from build123d import *

# Parameters (mm, degrees)
BOSS_EXTRUDE3_DEPTH  = 10
SKETCH2_W            = 34
SKETCH2_H            = 17
SKETCH2_W_2          = 30
SKETCH2_H_2          = 13
BOSS_EXTRUDE4_DEPTH  = 5
SKETCH3_W            = 50
SKETCH3_H            = 120
BOSS_EXTRUDE5_DEPTH  = 50
CUT_EXTRUDE2_DEPTH   = 50
SKETCH5_W            = 50
SKETCH5_H            = 180
BOSS_EXTRUDE6_DEPTH  = 50
CUT_EXTRUDE3_DEPTH   = 346.480399988
SKETCH7_W            = 5
SKETCH7_H            = 300
BOSS_EXTRUDE7_DEPTH  = 70
SKETCH9_W            = 34
SKETCH9_H            = 17
SKETCH9_W_2          = 30
SKETCH9_H_2          = 13
BOSS_EXTRUDE8_DEPTH  = 5
SKETCH10_W           = 55.647662557
SKETCH10_H           = 60
BOSS_EXTRUDE9_DEPTH  = 35
SKETCH13_W           = 13
SKETCH13_H           = 30
SKETCH13_W_2         = 8.592805021
SKETCH13_H_2         = 26
BOSS_EXTRUDE11_DEPTH = 5
SKETCH14_R           = 8
BOSS_EXTRUDE12_DEPTH = 27
SKETCH16_R           = 8
BOSS_EXTRUDE13_DEPTH = 27
SKETCH17_R           = 12
BOSS_EXTRUDE14_DEPTH = 5
SKETCH18_R           = 12
BOSS_EXTRUDE15_DEPTH = 5


with BuildPart() as part:
    # Sketch1 → Boss-Extrude3 (new body)
    with BuildSketch(Plane(origin=(0, 0, 0), x_dir=(1, 0, 0), z_dir=(0, 1, 0))):
        Polygon((-100.4558, 255.209143206), (299.5442, 255.209143206), (299.5442, 0.092543206), (229.0884, 0.092543206), (229.0884, -44.790856794), (-30, -44.790856794), (-30, 0.092543206), (-100.4558, 0.092543206), align=None)
    extrude(amount=BOSS_EXTRUDE3_DEPTH)

    # Sketch2 → Boss-Extrude4 (add)
    # profile 1 of 2: a face of its own
    with BuildSketch(Plane(origin=(0, 10, 0), x_dir=(1, 0, 0), z_dir=(0, 1, 0))):
        with Locations((-13, -22.349156794)):
            Rectangle(SKETCH2_W, SKETCH2_H)
        with Locations((-13, -22.349156794)):
            Rectangle(SKETCH2_W_2, SKETCH2_H_2, mode=Mode.SUBTRACT)
    # profile 2 of 2: a face of its own
    with BuildSketch(Plane(origin=(0, 10, 0), x_dir=(1, 0, 0), z_dir=(0, 1, 0))):
        with Locations((212.0884, -22.349156794)):
            Rectangle(SKETCH2_W, SKETCH2_H)
        with Locations((212.0884, -22.349156794)):
            Rectangle(SKETCH2_W_2, SKETCH2_H_2, mode=Mode.SUBTRACT)
    extrude(amount=BOSS_EXTRUDE4_DEPTH)

    # Sketch3 → Boss-Extrude5 (add)
    with BuildSketch(Plane(origin=(0, 10, 0), x_dir=(1, 0, 0), z_dir=(0, 1, 0))):
        with Locations((99.5442, 15.209143206)):
            Rectangle(SKETCH3_W, SKETCH3_H)
    extrude(amount=BOSS_EXTRUDE5_DEPTH)

    # Sketch4 → Cut-Extrude2 (cut)
    with BuildSketch(Plane(origin=(124.5442, 0, 0), x_dir=(0, 0, -1), z_dir=(1, 0, 0))):
        Polygon((-44.790856794, 60), (75.209143206, 60), (-44.790856794, 0), align=None)
    extrude(amount=-CUT_EXTRUDE2_DEPTH, mode=Mode.SUBTRACT)

    # Sketch5 → Boss-Extrude6 (add)
    with BuildSketch(Plane(origin=(0, 10, 0), x_dir=(1, 0, 0), z_dir=(0, 1, 0))):
        with Locations((99.5442, 165.209143206)):
            Rectangle(SKETCH5_W, SKETCH5_H)
    extrude(amount=BOSS_EXTRUDE6_DEPTH)

    # Sketch6 → Cut-Extrude3 (cut, through all)
    with BuildSketch(Plane(origin=(124.5442, 0, 0), x_dir=(0, 0, -1), z_dir=(1, 0, 0))):
        Polygon((75.209143206, 60), (255.209143206, 60), (255.209143206, 30), align=None)
    extrude(amount=-CUT_EXTRUDE3_DEPTH, mode=Mode.SUBTRACT)

    # Sketch7 → Boss-Extrude7 (add)
    with BuildSketch(Plane(origin=(0, 0, 0), x_dir=(1, 0, 0), z_dir=(0, 1, 0))):
        with Locations((72.0442, 105.209143206)):
            Rectangle(SKETCH7_W, SKETCH7_H)
        Polygon((129.5442, 255.209143206), (124.5442, 255.209143206), (124.5442, -44.790856794), (164.5442, -44.790856794), (164.5442, 0), (129.5442, 0), align=None)
    extrude(amount=BOSS_EXTRUDE7_DEPTH)

    # Sketch9 → Boss-Extrude8 (add)
    with BuildSketch(Plane(origin=(0, 70, 0), x_dir=(1, 0, 0), z_dir=(0, 1, 0))):
        with Locations((141.5442, -24.790856794)):
            Rectangle(SKETCH9_W, SKETCH9_H)
        with Locations((141.5442, -24.790856794)):
            Rectangle(SKETCH9_W_2, SKETCH9_H_2, mode=Mode.SUBTRACT)
    extrude(amount=BOSS_EXTRUDE8_DEPTH)

    # Sketch10 → Boss-Extrude9 (add)
    with BuildSketch(Plane(origin=(129.5442, 0, 0), x_dir=(0, 0, -1), z_dir=(1, 0, 0))):
        with Locations((227.385311928, 40)):
            Rectangle(SKETCH10_W, SKETCH10_H)
    extrude(amount=BOSS_EXTRUDE9_DEPTH)

    # Sketch13 → Boss-Extrude11 (add)
    with BuildSketch(Plane(origin=(0, 70, 0), x_dir=(1, 0, 0), z_dir=(0, 1, 0))):
        with Locations((142.552716242, 240.209143206)):
            Rectangle(SKETCH13_W, SKETCH13_H)
        with Locations((142.756313732, 240.209143206)):
            Rectangle(SKETCH13_W_2, SKETCH13_H_2, mode=Mode.SUBTRACT)
    extrude(amount=BOSS_EXTRUDE11_DEPTH)

    # Sketch14 → Boss-Extrude12 (add)
    with BuildSketch(Plane.XZ):
        with Locations(Location((284.5442, -240.209143206, 0), (0, 0, 90))):
            Circle(SKETCH14_R)
    extrude(amount=BOSS_EXTRUDE12_DEPTH)

    # Sketch16 → Boss-Extrude13 (add)
    with BuildSketch(Plane.XZ):
        with Locations(Location((-85.4558, -240.209143206, 0), (0, 0, 90))):
            Circle(SKETCH16_R)
    extrude(amount=BOSS_EXTRUDE13_DEPTH)

    # Sketch17 → Boss-Extrude14 (add)
    with BuildSketch(Plane.XZ.offset(27)):
        with Locations(Location((284.5442, -240.209143206, 0), (0, 0, 270))):
            Circle(SKETCH17_R)
    extrude(amount=BOSS_EXTRUDE14_DEPTH)

    # Sketch18 → Boss-Extrude15 (add)
    with BuildSketch(Plane.XZ.offset(27)):
        with Locations(Location((-85.4558, -240.209143206, 0), (0, 0, 270))):
            Circle(SKETCH18_R)
    extrude(amount=BOSS_EXTRUDE15_DEPTH)


solid = part.part
Work out the finished part from the listing and answer in its coordinate system (mm). A direction names the side the tool comes from. Coordinates: 2 decimals unless noted, no trailing zeros. Order: outer loops, then holes, each group sorted by start corner. A loop starts at its lowest first (then second) coordinate and runs counter-clockwise, first axis right, second up. Notation, with made-up numbers: (45.5, 88.25) - (72.5, 88.25) arc R36 cw to (72.5, 127.25) - close; hole circle Ø9 at (83, 16). An arc over 180 degrees is marked (long way). Put each result on its own line as item: value. Start each with the question number.
1) Find section D-D (x = -56.5). Give the vertices of the cut face in (y, z), plus the area to 3 significant figures.
2) Find the intervals of material crossed by line 1 (X direction, y = 63, z = -127); line 2 (X direction, y = 42, z = -173); line 3 (Y direction, x = 198, z = -180.5), in increasing order. Write a range as from..to.
3) For faces 4 (the cylindrical face through (279.14, -13.31, -246.11)), 5 (the flat face through (-13, 10, 22)), 6 (the flat face through (212, 15, 15)), 7 (the flat face through (265, 5, -0.093)), determine the directions among +Z, -Z, +X, -X, +Y, -Y from which every point of the face is accessible in a straight line to the end or side of a thin tool.
4) Find section A-A (x = -8.5). Give the vertices of the cut face in (y, z), plus the area to 3 significant figures.
5) Find section C-C (y = 49.5). Give the vertices of the cut face in (x, z).
6) Find section B-B (z = -105). Give the vertices of the cut face in (x, y), plus the area to 3 significant figures.
7) For a pull along X with two mould halves and no side action, classify faces 1 (the flat face through (113, 21, -255.209)), 2 (the flat face through (141, 70, 25)), 3 (the flat face through (164.544, 40, -227)) as released by +X, released by -X, zero draft, split by the parting line, or undercut.
8) Flat-ended cylindrical pins translate along their axes: pin 1 (3 mm diameter, centred on x = 73, z = -181.5, fed in from -Y); pin 2 (3 mm diameter, centred on x = 79.5, z = -100, fed in from +Y); pin 3 (6 mm diameter, centred on x = -32, z = -38.5, fed in from +Y). Find the tip coordinate at first contact, or state that the pin passes through.
Results list:
1. outline: (0, -255.21) - (10, -255.21) - (10, -0.09) - (0, -0.09) - close
1. area: 2,550 mm^2
2. line 1: x = 69.54..74.54, 124.54..129.54
2. line 2: x = 69.54..129.54
2. line 3: y = 0..10
3. face 4: none
3. face 5: +Y
3. face 6: +Z, -Z, +X, +Y
3. face 7: +Z, +X, +Y, -Y
4. outline: (0, -255.21) - (10, -255.21) - (10, 13.85) - (15, 13.85) - (15, 15.85) - (10, 15.85) - (10, 28.85) - (15, 28.85) - (15, 30.85) - (10, 30.85) - (10, 44.79) - (0, 44.79) - close
4. area: 3,020 mm^2
5. outline: (69.54, -255.21) - (74.54, -255.21) - (74.54, -138.21) - (124.54, -138.21) - (124.54, -255.21) - (164.54, -255.21) - (164.54, -199.56) - (129.54, -199.56) - (129.54, 0) - (164.54, 0) - (164.54, 44.79) - (124.54, 44.79) - (124.54, -54.21) - (74.54, -54.21) - (74.54, 44.79) - (69.54, 44.79) - close
6. outline: (-100.46, 0) - (299.54, 0) - (299.54, 10) - (129.54, 10) - (129.54, 70) - (124.54, 70) - (124.54, 55.03) - (74.54, 55.03) - (74.54, 70) - (69.54, 70) - (69.54, 10) - (-100.46, 10) - close
6. area: 6,850 mm^2
7. face 1: zero draft
7. face 2: undercut
7. face 3: released by +X
8. pin 1: stops at y = 0
8. pin 2: stops at y = 56.12
8. pin 3: stops at y = 10
